Input: part model. Units: mm. Frame: model coordinates. Coordinates: 2 decimals unless noted, no trailing zeros. Loops run counter-clockwise (first coordinate to the right, second up) from the corner with the lowest first, then second, coordinate; pieces in that order, holes last. Notation, with made-up numbers: (55, -11.5) -> (90, -11.5) arc R7 cw to (90, -2.5) -> close; hole circle Ø2 at (64, -12). An arc over 180 degrees is marked (long way). Answer as a JSON object with one key per item and string values.
from build123d import *

# Parameters (mm, degrees)
F2_DEPTH  = 0.4
F2_FACE_W = 0.96
F2_FACE_H = 0.4


with BuildPart() as f2:
    # F1 (on Top) → F2 (new body)
    with BuildSketch(Plane.XY):
        Polygon((-75, 84.52), (-75, 85), (-75, 85.48), (-76, 85.48), (-76, 84.52), align=None)
    extrude(amount=F2_DEPTH)

    # F3: sweep along a path in F1
    with BuildLine(Plane.XY) as f3_path:
        Line((-75, 85), (75, 85))
        Line((75, 85), (75, 65))
        Line((75, 65), (-75, 65))
        Line((-75, 65), (-75, 45))
        Line((-75, 45), (75, 45))
        Line((75, 45), (75, 25))
        Line((75, 25), (-75, 25))
        Line((-75, 25), (-75, 5))
        Line((-75, 5), (75, 5))
        Line((75, 5), (75, -15))
        Line((75, -15), (-75, -15))
        Line((-75, -15), (-75, -35))
        Line((-75, -35), (75, -35))
        Line((75, -35), (75, -55))
        Line((75, -55), (-75, -55))
        Line((-75, -55), (-75, -75))
        Line((-75, -75), (75, -75))
    # F2_face (on face) → F3 (sweep)
    with BuildSketch(Plane(origin=(-75, 85, 0.2), x_dir=(0, 1, 0), z_dir=(1, 0, 0))):
        Rectangle(F2_FACE_W, F2_FACE_H)
    sweep(path=f3_path.line, transition=Transition.RIGHT)


solid = f2.part
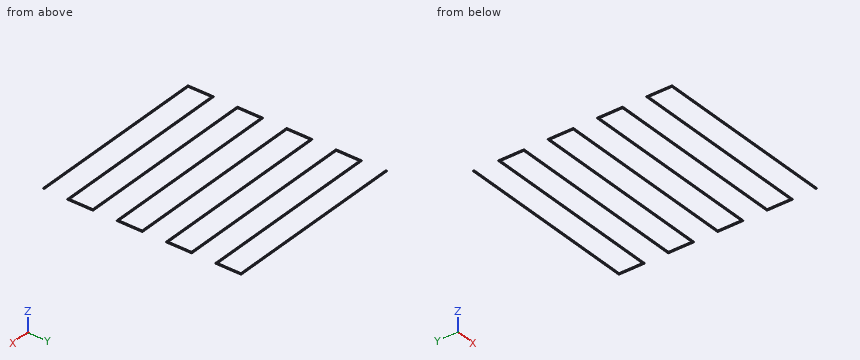
1. Line query: line 1 along X through (y, z) = (42.5, 0.35); line 2 along X through (y, z) = (-66.5, 0.1). Output: solid intervals per line, ascending.
Reply:
{"line 1": "x = 74.52 to 75.48", "line 2": "x = -75.48 to -74.52"}
2. Section query A-A (x = -35). Count the separate pieces of the cut face and the enclosed holes in it, plus the area to 3 significant figures.
Reply:
{"separate pieces": "9", "enclosed holes": "0", "area": "3.46 mm2"}
3. Pin query (flat end, axial travel): P1, Ø6, axis at x = 22, y = -9.5, coming from the -Z side. Return the tip coordinate at first contact, or that it passes through.
Reply:
{"P1": "passes through"}
4. Section query B-B (y = 41). Return loops of the section in (x, z), plus the area to 3 significant figures.
Reply:
{"outline": "(74.52, 0) -> (75.48, 0) -> (75.48, 0.4) -> (74.52, 0.4) -> close", "area": "0.384 mm2"}
